Job drawing, mm, ordinate dimensions from the low corner. One solid piece. A direction names the side the tool comes from. Give positions to 0.01 mm unless a question says otherwise; leave off trailing zeros. Write each loop counter-clockwise with the first axis right and the second up, starting at its lowest first coordinate (ties: lowest second). Pieces come first, ordered by that corner, then holes. Notation, with made-up numbers: (36.5, -3) - (51.5, -3) arc R23 cw to (51.5, 34) - close; hole circle Ø6 at (-14, -11). An arc over 180 degrees is marked (long way). Answer in a Markdown table with one row per item. Add a question column.
1. Band-saw the part on A-A on y = 11. Write the cut outline in (x, z), plus the area to 3 significant figures.
2. Probe line 1 along Z through (x, y) = (16.7, 11); line 2 along Y through (x, z) = (11, 11.75); line 3 along Z through (x, y) = (14.25, 19.5). List the from-to ranges inside material, lowest first.
3. Drop flat-ended pins along their axis: pin 1 Ø5 at (x, z) = (11, 14) entering from +Y; pin 2 Ø3 at (x, y) = (17.5, 4) entering from +Z; pin 3 Ø4 at (y, z) = (8, 3.5) entering from +X; pin 4 Ø9 at (x, y) = (11, 11) entering from +Z. Give the stop position or say it passes through.
4. Band-saw the part on C-C on z = 14. Write the cut outline in (x, y), plus the area to 3 significant figures.
5. Pull direction Z, two halves, no side cores. Call the marked faces 1, 2 and 3: released by +Z, released by -Z, zero draft, split by the parting line, or undercut.
6. Which spindle directions (+Z, -Z, +X, -X, +Y, -Y) get a long thin tool onto all of the face, cutting with end or side? Do the marked faces 4, 5 and 6. Say none if no direction does.
7. Band-saw the part on B-B on x = 11.75. Write the cut outline in (y, z), plus the area to 3 significant figures.
8. Band-saw the part on D-D on x = 17.25. Write the cut outline in (y, z), plus the area to 3 significant figures.
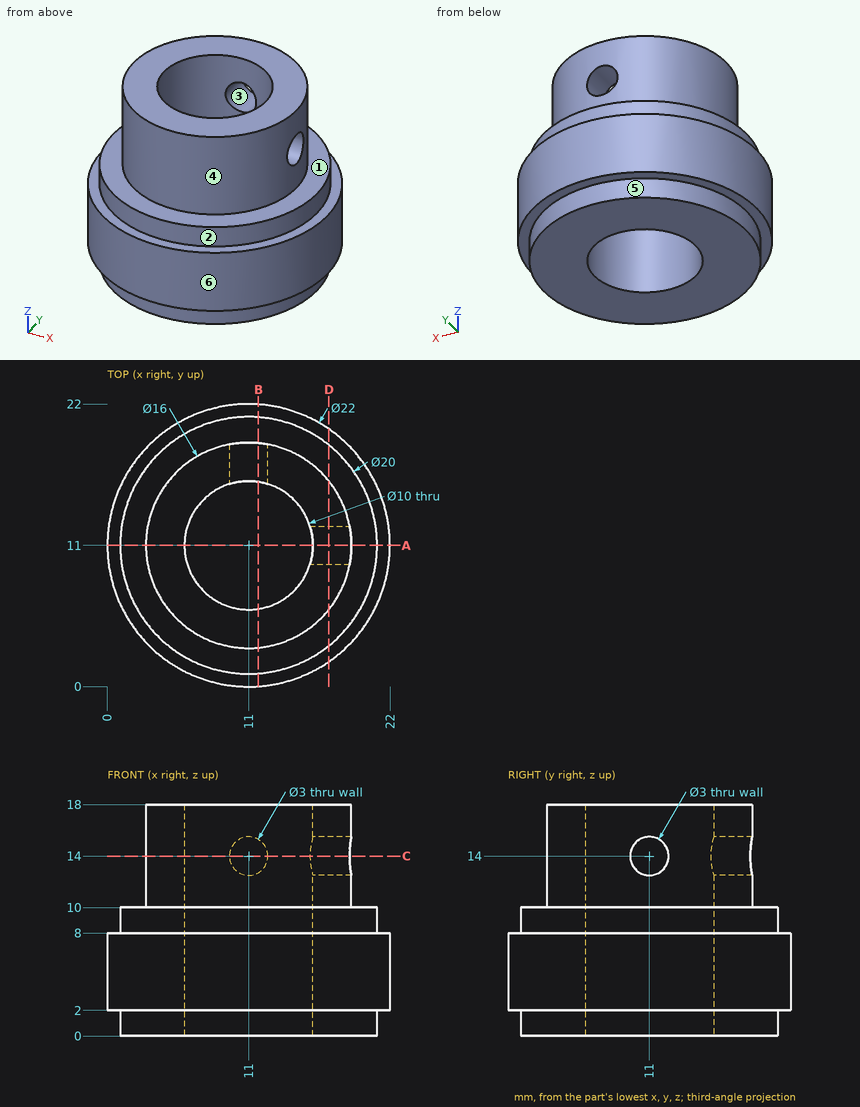
Values:
| question | item | result |
|---|---|---|
| 1 | outline | (0, 2) - (1, 2) - (1, 0) - (6, 0) - (6, 18) - (3, 18) - (3, 10) - (1, 10) - (1, 8) - (0, 8) - close; (16, 0) - (21, 0) - (21, 2) - (22, 2) - (22, 8) - (21, 8) - (21, 10) - (19, 10) - (19, 12.5) - (16, 12.5) - close; (16, 15.5) - (19, 15.5) - (19, 18) - (16, 18) - close |
| 1 | area | 151 mm² |
| 2 | line 1 | z = 0 to 12.5, 15.5 to 18 |
| 2 | line 2 | y = 3 to 6, 16 to 19 |
| 2 | line 3 | z = 0 to 10 |
| 3 | pin 1 | stops at y = 19 |
| 3 | pin 2 | stops at z = 10 |
| 3 | pin 3 | stops at x = 21.95 |
| 3 | pin 4 | passes through |
| 4 | outline | (9.5, 15.77) - (9.5, 18.86) arc R8 ccw (long way) to (18.86, 9.5) - (15.77, 9.5) arc R5 cw (long way) to start; (12.5, 15.77) arc R5 cw to (15.77, 12.5) - (18.86, 12.5) arc R8 ccw to (12.5, 18.86) - close |
| 4 | area | 104 mm² |
| 5 | face 1 | released by +Z |
| 5 | face 2 | zero draft |
| 5 | face 3 | undercut |
| 6 | face 4 | +Z |
| 6 | face 5 | -Z |
| 6 | face 6 | +Z, -Z |
| 7 | outline | (0.03, 2) - (1.03, 2) - (1.03, 0) - (6.06, 0) - (6.06, 18) - (3.04, 18) - (3.04, 10) - (1.03, 10) - (1.03, 8) - (0.03, 8) - close; (15.94, 0) - (20.97, 0) - (20.97, 2) - (21.97, 2) - (21.97, 8) - (20.97, 8) - (20.97, 10) - (18.96, 10) - (18.96, 12.7) - (15.94, 12.7) - close; (15.94, 15.3) - (18.96, 15.3) - (18.96, 18) - (15.94, 18) - close |
| 7 | area | 153 mm² |
| 8 | outline | (1.95, 2) - (3.19, 2) - (3.19, 0) - (18.81, 0) - (18.81, 2) - (20.05, 2) - (20.05, 8) - (18.81, 8) - (18.81, 10) - (15.99, 10) - (15.99, 18) - (6.01, 18) - (6.01, 10) - (3.19, 10) - (3.19, 8) - (1.95, 8) - close; hole circle Ø3 at (11, 14) |
| 8 | area | 244 mm² |
